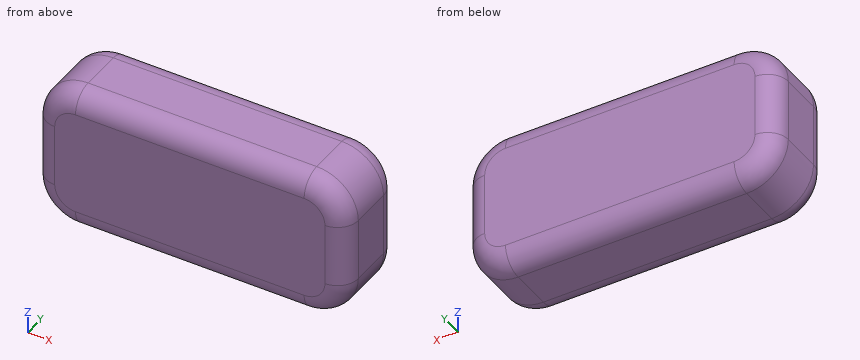
Autodesk Inventor part; units mm, degrees
ref_plane "YZ Plane" through (0, 0, 0) normal (1, 0, 0) x (0, 1, 0)
ref_plane "XZ Plane" through (0, 0, 0) normal (0, 1, 0) x (-1, 0, 0)
ref_plane "XY Plane" through (0, 0, 0) normal (0, 0, 1) x (1, 0, 0)
sketch "Sketch1" plane through (0, 0, 0) normal (0, 1, 0) x (-1, 0, 0)
  line L0 (-47.625, -22.225) -> (47.625, -22.225)
  line L1 (47.625, -22.225) -> (47.625, 22.225)
  line L2 (47.625, 22.225) -> (-47.625, 22.225)
  line L3 (-47.625, 22.225) -> (-47.625, -22.225)
  line L4 (-47.625, -22.225) -> (47.625, 22.225) construction
  line L5 (47.625, -22.225) -> (-47.625, 22.225) construction
  point P0 (0, 0)
  dimension "d0" = 95.25
  dimension "d1" = 44.45
extrude "Extrusion1" add sketch "Sketch1" along normal blind 25.4
fillet "Fillet1" radius 12.7 4 edges at (-47.625, 12.7, 22.225) (47.625, 12.7, 22.225) (47.625, 12.7, -22.225) (-47.625, 12.7, -22.225)
fillet "Fillet2" radius 6.35 16 edges at (43.9053, 25.4, 18.5053) (47.625, 25.4, 0) (43.9053, 25.4, -18.5053) (0, 25.4, -22.225) (-43.9053, 25.4, -18.5053) (-47.625, 25.4, 0) (-43.9053, 25.4, 18.5053) (0, 25.4, 22.225) (43.9053, 0, 18.5053) (47.625, 0, 0) (43.9053, 0, -18.5053) (0, 0, -22.225) (-43.9053, 0, -18.5053) (-47.625, 0, 0) (-43.9053, 0, 18.5053) (0, 0, 22.225)
properties part number "am-3277"
Source: CAD feature listing. Evaluate the final solid. Frame: model axes, mm. Round coordinates to 2 decimals unless told otherwise and drop trailing zeros. Write each loop counter-clockwise with the first axis right and the second up, starting at its lowest first coordinate (ties: lowest second). Pieces come first, ordered by that corner, then holes. Notation, with made-up numbers: M 87.5,31 L 92.5,31 A23 cw 92.5,66 Z; hole C -22.5,30 d8. An arc over 180 degrees is marked long. One line per item, written item: value. Start each with the question number.
Item 1: Ray query, L1, parallel to X at y = 12.75, z = -10; L2, parallel to Y at x = -12, z = -16; L3, parallel to X at y = 20.25, z = 14. Return the intervals inside material, ascending. Write a range as from..to.
Item 2: Section query A-A (x = -9). Return the cut outline in (y, z) (3 decimals).
Item 3: Pin query (flat end, axial travel): pin 1 (10 mm diameter, centred on y = 4.5, z = -17, fed in from +X); pin 2 (2 mm diameter, centred on y = 15.5, z = -16.5, fed in from +X); pin 3 (2 mm diameter, centred on y = 21.5, z = 17.5, fed in from +X). Return the tip coordinate at first contact, or that it passes through.
Item 4: Section query B-B (y = 12.25). Return the cut outline in (x, z) (3 decimals), plus the area to 3 significant figures.
Result set:
1. L1: x = -47.62..47.62
1. L2: y = 0..25.4
1. L3: x = -46.69..46.69
2. outline: M 0,-15.875 A6.35 ccw 6.35,-22.225 L 19.05,-22.225 A6.35 ccw 25.4,-15.875 L 25.4,15.875 A6.35 ccw 19.05,22.225 L 6.35,22.225 A6.35 ccw 0,15.875 Z
3. pin 1: stops at x = 47.32
3. pin 2: stops at x = 46.13
3. pin 3: stops at x = 45.08
4. outline: M -47.625,-9.525 A12.7 ccw -34.925,-22.225 L 34.925,-22.225 A12.7 ccw 47.625,-9.525 L 47.625,9.525 A12.7 ccw 34.925,22.225 L -34.925,22.225 A12.7 ccw -47.625,9.525 Z
4. area: 4,100 mm²
